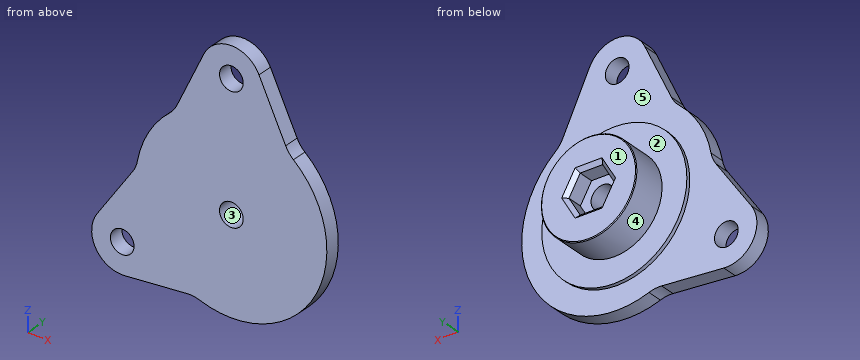
```python
from build123d import *

# Parameters (mm, degrees)
CUT_EXTRUDE1_DEPTH  = 5
SKETCH4_R           = 3.1
CUT_EXTRUDE2_DEPTH  = 39.026306684
CHAMFER1_SIZE       = 0.2
BOSS_EXTRUDE1_START = 4
SKETCH6_R           = 3.1
BOSS_EXTRUDE1_DEPTH = 4
CIRPATTERN1_COUNT   = 2
CIRPATTERN1_ANGLE   = 120
FILLET2_R           = 8
CHAMFER2_SIZE       = 1


with BuildPart() as part:
    # Sketch2 → Revolve1 (revolve)
    with BuildSketch(Plane.XY, mode=Mode.PRIVATE) as revolve1_sk:
        Polygon((0, 0), (25, 0), (25, 4), (19, 4), (19, 5), (12.5, 5), (12.5, 14), (0, 14), align=None)
    revolve(revolve1_sk.sketch.rotate(Axis((0, 0, 0), (0, 1, 0)), 90), axis=Axis((0, 0, 0), (0, 1, 0)))

    # Sketch3 → Cut-Extrude1 (cut)
    with BuildSketch(Plane(origin=(0, 14, 0), x_dir=(1, 0, 0), z_dir=(0, 1, 0))):
        Polygon((5.888972746, 0), (2.944486373, 5.1), (-2.944486373, 5.1), (-5.888972746, 0), (-2.944486373, -5.1), (2.944486373, -5.1), align=None)
    extrude(amount=-CUT_EXTRUDE1_DEPTH, mode=Mode.SUBTRACT)

    # Sketch4 → Cut-Extrude2 (cut, through all)
    with BuildSketch(Plane(origin=(0, 0, 0), x_dir=(1, 0, 0), z_dir=(0, 1, 0))):
        with Locations(Location((0, 0, 0), (0, 0, 90))):
            Circle(SKETCH4_R)
    extrude(amount=CUT_EXTRUDE2_DEPTH, mode=Mode.SUBTRACT)

    # Chamfer1
    chamfer1_edges = [part.edges().sort_by_distance(p)[0] for p in [
        (0, 14, 12.5),
    ]]
    chamfer(chamfer1_edges, length=CHAMFER1_SIZE)

    # Sketch6 → Boss-Extrude1 (add)
    with BuildSketch(Plane(origin=(0, 0, 0), x_dir=(1, 0, 0), z_dir=(0, 1, 0)).offset(BOSS_EXTRUDE1_START)):
        with BuildLine():
            ThreePointArc((15, -20), (0, -25), (-15, -20))
            Line((-15, -20), (-7.231608683, -36.421086941))
            ThreePointArc((-7.231608683, -36.421086941), (0, -41), (7.231608683, -36.421086941))
            Line((7.231608683, -36.421086941), (15, -20))
        make_face()
        with Locations(Location((0, -33, 0), (0, 0, 270))):
            Circle(SKETCH6_R, mode=Mode.SUBTRACT)
    boss_extrude1 = extrude(amount=-BOSS_EXTRUDE1_DEPTH)

    # CirPattern1: Boss-Extrude1 ×2 about axis
    cirpattern1_axis = Axis((0, 0, 0), (0, -1, 0))
    for i in range(1, CIRPATTERN1_COUNT):
        add(boss_extrude1.rotate(cirpattern1_axis, i * CIRPATTERN1_ANGLE / (CIRPATTERN1_COUNT - 1)))

    # Fillet2
    fillet2_edges = [part.edges().sort_by_distance(p)[0] for p in [
        (-15, 2, 20),
        (15, 2, 20),
        (-9.820508076, 2, -22.990381057),
        (-24.820508076, 2, 2.990381057),
    ]]
    fillet(fillet2_edges, radius=FILLET2_R)

    # Chamfer2
    chamfer2_edges = [part.edges().sort_by_distance(p)[0] for p in [
        (4.416729559, 14, 2.55),
        (4.416729559, 14, -2.55),
        (0, 14, -5.1),
        (-4.416729559, 14, -2.55),
        (-4.416729559, 14, 2.55),
        (0, 14, 5.1),
    ]]
    chamfer(chamfer2_edges, length=CHAMFER2_SIZE)


solid = part.part
```
Model file for the job. Use its own axes, mm. Face numbers are marked on the shaded views. A direction names the side the tool comes from. Coordinates: 2 decimals unless noted, no trailing zeros. Write each loop counter-clockwise with the first axis right and the second up, starting at its lowest first coordinate (ties: lowest second). Pieces come first, ordered by that corner, then holes. Notation, with made-up numbers: (1, -0.5) - (30, -0.5) arc R16 ccw to (30, 7.5) - close; hole circle Ø5 at (19.5, 47). An arc over 180 degrees is marked (long way). Use a Markdown table: item, result. Add a question column.
Item 1: Drop flat-ended pins along their axis: pin 1 (1 mm diameter, centred on x = -20.5, z = 10, fed in from +Y); pin 2 (2 mm diameter, centred on x = -27, y = 6, fed in from -Z); pin 3 (1.2 mm diameter, centred on x = -1, y = 11, fed in from +Z); pin 4 (8 mm diameter, centred on y = 3.5, z = 34.5, fed in from +X). Give the stop position or say it passes through.
Item 2: Two-plate mould, pull along X, no slides. Class the marked faces 3, 4 and 5: pulls with the +X half, pulls with the -X half, needs draft (parallel to the pull), parting line crosses it, or undercut.
Item 3: 3-axis set-ups, long thin cutter, end or side, ignore diameter. For the marked faces 1 and 2: which of +Z, -Z, +X, -X, +Y, -Y reach the whole face in a straight line?
Item 4: Band-saw the part on D-D, the plane y = 7.25. Write the cut outline in (x, z), and give its area (3 significant figures).
Item 5: Drill centre lines: line 1 along X through (y, z) = (5.25, 0); line 2 along Y through (x, z) = (9, 22); line 3 along X through (y, z) = (2.5, 0). Where is each one in solid material? Low to high.
Item 6: Band-saw the part on C-C, the plane y = 2.5. Write the cut outline in (x, z), and give its area (3 significant figures).
Item 7: Band-saw the part on B-B, the plane z = 33. Write the cut outline in (x, y), and give its area (3 significant figures).
Item 8: Band-saw the part on A-A, the plane x = 0. Write the cut outline in (y, z), and give its area (3 significant figures).
A:
| question | item | result |
|---|---|---|
| 1 | pin 1 | stops at y = 4 |
| 1 | pin 2 | passes through |
| 1 | pin 3 | stops at z = 12.49 |
| 1 | pin 4 | stops at x = 10.03 |
| 2 | face 3 | undercut |
| 2 | face 4 | parting line crosses it |
| 2 | face 5 | needs draft |
| 3 | face 1 | +Z, -Z, +X, -X, +Y |
| 3 | face 2 | +Y |
| 4 | outline | circle Ø25 at (0, 0); hole circle Ø6.2 at (0, 0) |
| 4 | area | 461 mm² |
| 5 | line 1 | x = -12.5 to -3.1, 3.1 to 12.5 |
| 5 | line 2 | y = 0 to 4 |
| 5 | line 3 | x = -26.89 to -3.1, 3.1 to 25 |
| 6 | outline | (-35.16, -11.95) arc R8 ccw to (-27.93, -24.47) - (-11.65, -23.14) arc R8 cw to (-8.33, -23.57) arc R25 ccw to (16.25, 19) arc R8 cw to (14.21, 21.66) - (7.23, 36.42) arc R8 ccw to (-7.23, 36.42) - (-14.21, 21.66) arc R8 cw to (-16.25, 19) arc R25 ccw to (-24.58, 4.57) arc R8 cw to (-25.87, 1.48) - close; hole circle Ø6.2 at (-28.58, -16.5); hole circle Ø6.2 at (0, 0); hole circle Ø6.2 at (0, 33) |
| 6 | area | 2,490 mm² |
| 7 | outline | (-8.85, 0) - (-3.1, 0) - (-3.1, 4) - (-8.85, 4) - close; (3.1, 0) - (8.85, 0) - (8.85, 4) - (3.1, 4) - close |
| 7 | area | 46.0 mm² |
| 8 | outline | (0, -25) - (4, -25) - (4, -19) - (5, -19) - (5, -12.5) - (13.8, -12.5) - (14, -12.3) - (14, -6.1) - (13, -5.1) - (9, -5.1) - (9, -3.1) - (0, -3.1) - close; (0, 3.1) - (9, 3.1) - (9, 5.1) - (13, 5.1) - (14, 6.1) - (14, 12.3) - (13.8, 12.5) - (5, 12.5) - (5, 19) - (4, 19) - (4, 29.9) - (0, 29.9) - close; (0, 36.1) - (4, 36.1) - (4, 41) - (0, 41) - close |
| 8 | area | 394 mm² |
